The listing builds one solid part. Answer for the finished solid, in the listing's coordinates (mm). A direction names the side the tool comes from. Coordinates: 2 decimals unless noted, no trailing zeros. Loops run counter-clockwise (first coordinate to the right, second up) from the corner with the lowest first, then second, coordinate; pieces in that order, holes last. Notation, with made-up numbers: (47, 18) - (104, 18) arc R17 ccw to (104, 42) - close; hole circle Ø10 at (-10, 84). An arc over 180 degrees is marked (long way). Return JSON: item names as keys, results as strings. Group by question number.
1. Section A-A (z = -18) is taken. Write down the section's boundary in (x, y).
2. Section B-B (z = -5) is taken. Write down the section's boundary in (x, y), and give its area (3 significant figures).
3. Each of these flat-tipped pins is pushed along its axis until it touches: P1, Ø2, axis at x = -16, z = -33, coming from the -Y side; P2, Ø2, axis at x = 0, y = 27.9, coming from the -Z side; P3, Ø12, axis at x = -23.5, z = -20.5, coming from the -Y side. Where does it stop, or does it pass through?
4. The mould has two halves that part along Y. Classify faces 4 (the face through (16.88, 5.32, 4.29)), 5 (the face through (-1.8, -22.5, -49.8)), 6 (the face through (-16, 20, -54.8)): pulls with the +Y half, pulls with the -Y half, needs draft (parallel to the pull), parting line crosses it, or undercut.
5. Which of the six approach directions +Z, -Z, +X, -X, +Y, -Y give full straight-line access (tool end or side, diameter ignored) to faces 1 (the face through (30.37, 1.34, -39.89)), 2 (the face through (-7, -9, 0)), 3 (the face through (5.506, -24.796, -52.265))?
6. Find the intervals of material crossed by line 1 along Y through (x, z) = (0, -53.05); line 2 along Y through (x, z) = (0, 6); line 3 along X through (y, z) = (-2, -33), in increasing order.
```python
from build123d import *

# Parameters (mm, degrees)
ESQUISSE1_R                     = 17.7
ESQUISSE1_R_2                   = 12.7
BOSS_EXTRU_1_DEPTH              = 8.7
ESQUISSE2_R                     = 30.4
ESQUISSE2_R_2                   = 11.2
BOSS_EXTRU_2_DEPTH              = 49.8
CHANFREIN1_SIZE                 = 25.4
CHANFREIN1_SIZE2                = 12.699971641
CHANFREIN3_SIZE                 = 11.200084029
CHANFREIN3_SIZE_2               = 49.8
F_41_0_096_DIAMETER_HOLE1_D     = 2.4384
F_41_0_096_DIAMETER_HOLE1_DEPTH = 5
F_41_0_096_DIAMETER_HOLE1_TIP   = 0.732569267
SKETCH5_R                       = 30.4
SKETCH5_R_2                     = 25.4
BOSS_EXTRUDE1_DEPTH             = 5


# Read off the part's stored shape, not the designer's step: AdvancedHole1
with BuildPart() as part:
    # Esquisse1 → Boss.-Extru.1 (new body)
    with BuildSketch(Plane.XY):
        Circle(ESQUISSE1_R)
        Circle(ESQUISSE1_R_2, mode=Mode.SUBTRACT)
    extrude(amount=BOSS_EXTRU_1_DEPTH)

    # Esquisse2 → Boss.-Extru.2 (add)
    with BuildSketch(Plane(origin=(0, 0, 0), x_dir=(-1, 0, 0), z_dir=(0, 0, -1))):
        Circle(ESQUISSE2_R)
        Circle(ESQUISSE2_R_2, mode=Mode.SUBTRACT)
    extrude(amount=BOSS_EXTRU_2_DEPTH)

    # Chanfrein1
    chanfrein1_edges = [part.edges().sort_by_distance(p)[0] for p in [
        (30.4, 0, 0),
    ]]
    chanfrein1_side = [part.faces().sort_by_distance(p)[0] for p in [
        (30.4, 0, -24.9),
    ]]
    chamfer(chanfrein1_edges, length=CHANFREIN1_SIZE, length2=CHANFREIN1_SIZE2, reference=chanfrein1_side[0])

    # Chanfrein3
    # the kernel refuses this chamfer: 49.8, 11.200084029 mm, written as the material it takes off along each edge
    with BuildSketch(Plane(origin=(0, 0, -49.8), x_dir=(-1, 0, 0), z_dir=(0, -1, 0))) as chanfrein3_piece_1:
        Polygon((11.2 + CHANFREIN3_SIZE, 0), (11.2, -CHANFREIN3_SIZE_2), (11.2, 0), align=None)
    revolve(axis=Axis((0, 0, -49.8), (0, 0, -1)), mode=Mode.SUBTRACT)

    # #41 (0.096) Diameter Hole1
    with Locations(Plane.XY.offset(8.7)):
        with Locations((-15.2, 0), (15.2, 0)):
            Hole(F_41_0_096_DIAMETER_HOLE1_D / 2, depth=F_41_0_096_DIAMETER_HOLE1_DEPTH)
            with Locations((0, 0, -(F_41_0_096_DIAMETER_HOLE1_DEPTH + F_41_0_096_DIAMETER_HOLE1_TIP / 2))):  # 118° drill point
                Cone(0, F_41_0_096_DIAMETER_HOLE1_D / 2, F_41_0_096_DIAMETER_HOLE1_TIP, mode=Mode.SUBTRACT)

    # Sketch5 → Boss-Extrude1 (add)
    with BuildSketch(Plane(origin=(0, 0, -49.8), x_dir=(-1, 0, 0), z_dir=(0, 0, -1))):
        Circle(SKETCH5_R)
        Circle(SKETCH5_R_2, mode=Mode.SUBTRACT)
    extrude(amount=BOSS_EXTRUDE1_DEPTH)

    # AdvancedHole1 outline → AdvancedHole1 (revolve, cut)
    with BuildSketch(Plane.XZ.offset(-27.9)):
        Polygon((1.2192, -54.8), (1.2192, -49.72), (0, -48.987430733), (0, -54.8), align=None)
    advancedhole1 = revolve(axis=Axis((0, 27.9, 0), (0, 0, 1)), mode=Mode.SUBTRACT)

    # Mirror1: AdvancedHole1 across plane
    add(advancedhole1.mirror(Plane.ZX), mode=Mode.SUBTRACT)


solid = part.part
```
The answers:
{
 "1": {"outline": "circle Ø53.4 at (0, 0); hole circle Ø30.5 at (0, 0)"},
 "2": {"outline": "circle Ø40.4 at (0, 0); hole circle Ø24.65 at (0, 0)", "area": "805 mm2"},
 "3": {"P1": "stops at y = -26.44", "P2": "stops at z = -49.59", "P3": "stops at y = -23.14"},
 "4": {"face 4": "parting line crosses it", "face 5": "undercut", "face 6": "needs draft"},
 "5": {"face 1": "+Z, -Z", "face 2": "+Z", "face 3": "-Z"},
 "6": {"line 1": "y = -30.4 to -29.12, -26.68 to -25.4, 25.4 to 26.68, 29.12 to 30.4", "line 2": "y = -17.7 to -12.7, 12.7 to 17.7", "line 3": "x = -30.33 to -18.51, 18.51 to 30.33"}
}
